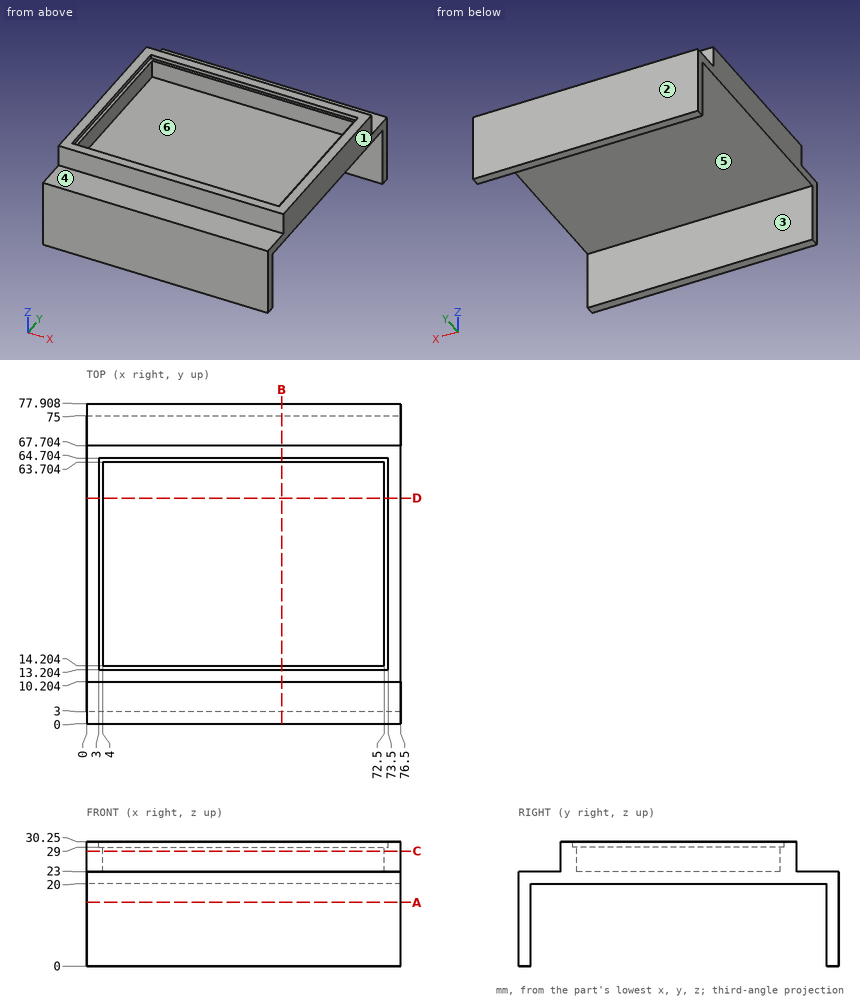
Drawing for the job (mm, zero at the part's lowest x, y, z). A direction names the side the tool comes from. Round coordinates to 2 decimals unless told otherwise and drop trailing zeros. Order: outer loops, then holes, each group sorted by start corner. A loop starts at its lowest first (then second) coordinate and runs counter-clockwise, first axis right, second up. Notation, with made-up numbers: (-20, 34.5) -> (-15, 34.5) arc R11 cw to (-15, 42.5) -> close; hole circle Ø7 at (-27, 54.5). An arc over 180 degrees is marked (long way). Write item = value, one per line. Start each with the question number.
(1) Cut at C-C, the plane z = 28. List the corners of the cut face in (x, y).
(2) Cut at D-D, the plane y = 55. List the corners of the cut face in (x, z).
(3) Cut at B-B, the plane x = 47.5. List the corners of the cut face in (y, z).
(4) Pin check, flat tips, straight feed: P1, Ø3, axis at x = 21.5, z = 27, coming from the +Y side; P2, Ø1.4, axis at x = 52.5, z = 29.5, coming from the -Y side; P3, Ø21.5, axis at x = 22.5, y = 52.5, coming from the -Z side. Stop position of each tip, or through.
(5) Probe line 1 (Y direction, x = 18, z = 9); line 2 (X direction, y = 50, z = 27); line 3 (Z direction, x = 3, y = 66.5). List the from-to ranges inside material, lowest first. Write a range as [from, to].
(6) Which spindle directions (+Z, -Z, +X, -X, +Y, -Y) get a long thin tool onto all of the face, cutting with end or side? Do the marked faces 4, 5 and 6. Say none if no direction does.
(7) Pull direction Y, two halves, no side cores. Call the marked faces 1, 2 and 3: released by +Y, released by -Y, zero draft, split by the parting line, or undercut.
(8) Cut at A-A, the plane z = 15.5. List the corners of the cut face in (x, y), then the cut area to 3 significant figures.
Model answer:
q1.outline = (0, 10.2) -> (76.5, 10.2) -> (76.5, 67.7) -> (0, 67.7) -> close; hole (4, 14.2) -> (72.5, 14.2) -> (72.5, 63.7) -> (4, 63.7) -> close
q2.outline = (0, 20) -> (76.5, 20) -> (76.5, 30.25) -> (73.5, 30.25) -> (73.5, 29) -> (72.5, 29) -> (72.5, 23) -> (4, 23) -> (4, 29) -> (3, 29) -> (3, 30.25) -> (0, 30.25) -> close
q3.outline = (0, 0) -> (3, 0) -> (3, 20) -> (75, 20) -> (75, 0) -> (77.91, 0) -> (77.91, 23) -> (67.7, 23) -> (67.7, 30.25) -> (64.7, 30.25) -> (64.7, 29) -> (63.7, 29) -> (63.7, 23) -> (14.2, 23) -> (14.2, 29) -> (13.2, 29) -> (13.2, 30.25) -> (10.2, 30.25) -> (10.2, 23) -> (0, 23) -> close
q4.P1 = 67.7
q4.P2 = 10.2
q4.P3 = 20
q5.line_1 = [0, 3], [75, 77.91]
q5.line_2 = [0, 4], [72.5, 76.5]
q5.line_3 = [20, 30.25]
q6.face_4 = +Z, +X, -X, -Y
q6.face_5 = -Z, +X, -X
q6.face_6 = +Z
q7.face_1 = zero draft
q7.face_2 = released by +Y
q7.face_3 = undercut
q8.outline = (0, 0) -> (76.5, 0) -> (76.5, 3) -> (0, 3) -> close; (0, 75) -> (76.5, 75) -> (76.5, 77.91) -> (0, 77.91) -> close
q8.area = 452 mm2
